from build123d import *

# Parameters (mm, degrees)
SKETCH1_W           = 22
SKETCH1_H           = 10
SKETCH1_R           = 1.5
BOSS_EXTRUDE1_DEPTH = 5
SKETCH4_W           = 6
SKETCH4_H           = 10
BOSS_EXTRUDE3_DEPTH = 13
CUT_EXTRUDE1_REACH  = 16
SKETCH5_R           = 1.5
FILLET1_R           = 2


with BuildPart() as part:
    # Sketch1 → Boss-Extrude1 (new body)
    with BuildSketch(Plane(origin=(0, 0, 0), x_dir=(1, 0, 0), z_dir=(0, 1, 0))):
        Rectangle(SKETCH1_W, SKETCH1_H)
        with Locations((-7, 0)):
            Circle(SKETCH1_R, mode=Mode.SUBTRACT)
        with Locations((7, 0)):
            Circle(SKETCH1_R, mode=Mode.SUBTRACT)
    extrude(amount=BOSS_EXTRUDE1_DEPTH)

    # Sketch4 → Boss-Extrude3 (add)
    with BuildSketch(Plane(origin=(0, 5, 0), x_dir=(1, 0, 0), z_dir=(0, 1, 0))):
        Rectangle(SKETCH4_W, SKETCH4_H)
    extrude(amount=BOSS_EXTRUDE3_DEPTH)

    # Sketch5 → Cut-Extrude1 (cut, up to next)
    with BuildSketch(Plane(origin=(3, 0, 0), x_dir=(0, 0, -1), z_dir=(1, 0, 0)), mode=Mode.PRIVATE) as cut_extrude1_sk1:
        with Locations((0, 13)):
            Circle(SKETCH5_R)
    cut_extrude1_tool1 = extrude(cut_extrude1_sk1.sketch, amount=-CUT_EXTRUDE1_REACH, mode=Mode.PRIVATE) & part.part
    add(cut_extrude1_tool1.solids().sort_by_distance((3, 13, 0))[0], mode=Mode.SUBTRACT)

    # Fillet1
    fillet1_edges = [part.edges().sort_by_distance(p)[0] for p in [
        (0, 18, -5),
        (0, 18, 5),
    ]]
    fillet(fillet1_edges, radius=FILLET1_R)


solid = part.part
Here's how the part is built. I have some questions about the finished solid (model axes, mm). A direction names the side the tool comes from. Coordinates: 2 decimals unless noted, no trailing zeros. Write each loop counter-clockwise with the first axis right and the second up, starting at its lowest first coordinate (ties: lowest second). Pieces come first, ordered by that corner, then holes.
1) If we section it at D-D (z = 2.25): List the corners of the cut face in (x, y) for me, plus the area to 3 significant figures.
Filled in:
outline: (-11, 0) - (11, 0) - (11, 5) - (3, 5) - (3, 18) - (-3, 18) - (-3, 5) - (-11, 5) - close
area: 188 mm2
2) Thinking about a two-plate mould opening in Z: for faces 4 (the face through (5.5, 2.46, -0.07)), 5 (the face through (0.04, 17.4, 4.43)), 6 (the face through (5, 5, 0)), which applies, +Z half, -Z half, draft (parallel to the pull), parting line (faces both ways), or undercut?
Filled in:
face 4: undercut
face 5: +Z half
face 6: draft
3) If we section it at B-B (x = -7): List the corners of the cut face in (y, z) for me, plus the area to 3 significant figures.
Filled in:
outline: (0, -5) - (5, -5) - (5, -1.5) - (0, -1.5) - close; (0, 1.5) - (5, 1.5) - (5, 5) - (0, 5) - close
area: 35.0 mm2
4) If we section it at C-C (x = -1): List the corners of the cut face in (y, z) for me.
Filled in:
outline: (0, -5) - (16, -5) arc R2 ccw to (18, -3) - (18, 3) arc R2 ccw to (16, 5) - (0, 5) - close; hole circle Ø3 at (13, 0)
5) Which directions (+Z, -Z, +X, -X, +Y, -Y) give clear straight access to the entire face, cutting with the end or side of a thin tool? Please do faces 1 (the face through (3, 11, 0)), 2 (the face through (-9, 5, 0)), 3 (the face through (-8.5, 2.46, -0.07)).
Filled in:
face 1: +Z, -Z, +X, +Y
face 2: +Z, -Z, -X, +Y
face 3: +Y, -Y
6) If I drill on line 1 (X direction, y = 2.95, z = 0); line 2 (Z direction, x = -7, y = 2.85); line 3 (Y direction, x = -8.75, z = -3.5), over which ranges is the centre line in solid material (lowest first)?
Filled in:
line 1: x = -11 to -8.5, -5.5 to 5.5, 8.5 to 11
line 2: z = -5 to -1.5, 1.5 to 5
line 3: y = 0 to 5
7) I'm going to push flat-ended pins straight in: pin 1 (5 mm diameter, centred on y = 13, z = 0, fed in from +X); pin 2 (3.5 mm diameter, centred on x = 7, z = 0, fed in from +Y); pin 3 (5 mm diameter, centred on y = 10, z = 1.5, fed in from -X). Where does each tip first touch, or does it pass through?
Filled in:
pin 1: stops at x = 3
pin 2: stops at y = 5
pin 3: stops at x = -3
8) If we section it at A-A (y = 13): List the corners of the cut face in (x, z) for me.
Filled in:
outline: (-3, -5) - (3, -5) - (3, -1.5) - (-3, -1.5) - close; (-3, 1.5) - (3, 1.5) - (3, 5) - (-3, 5) - close
